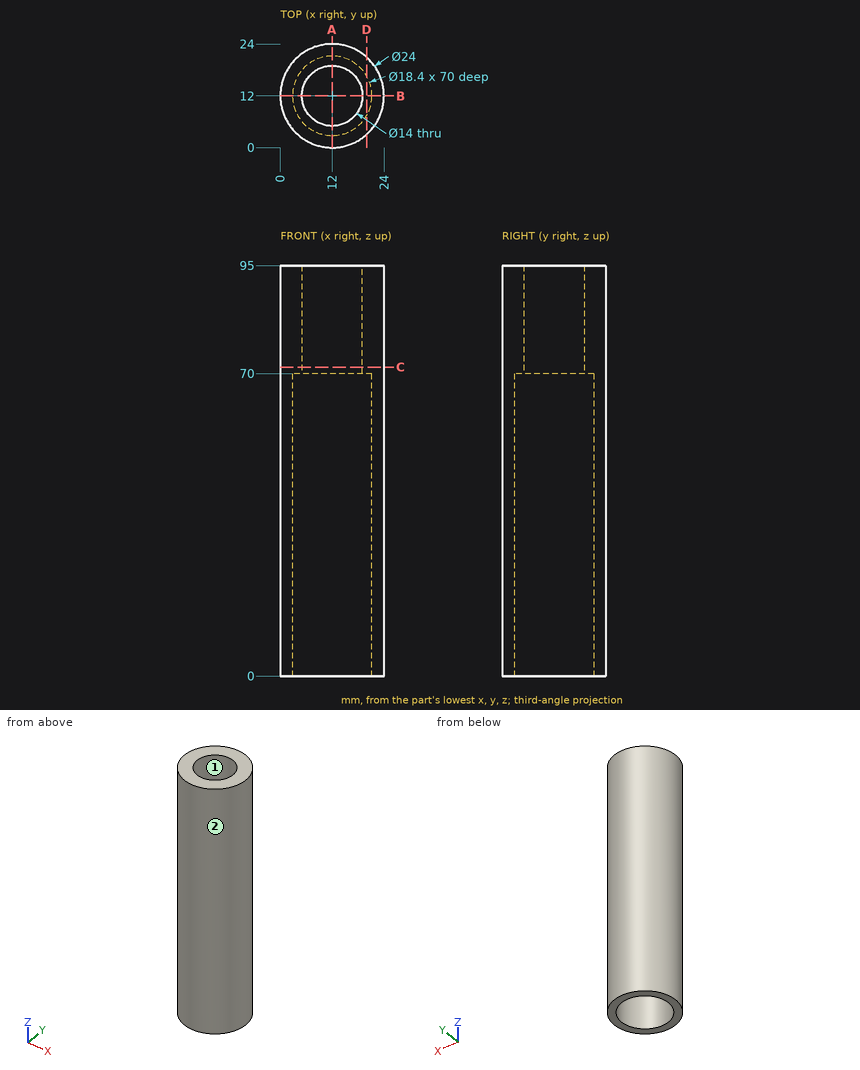
The drawing under review shows one solid part. Ordinate dimensions are in mm from its lowest x, y, z. Give positions to 0.01 mm unless a question says otherwise; leave off trailing zeros. Write each loop counter-clockwise with the first axis right and the second up, starting at its lowest first coordinate (ties: lowest second). Pieces come first, ordered by that corner, then holes. Notation, with made-up numbers: (13.25, 81) -> (48.25, 81) arc R32 ccw to (48.25, 113) -> close; hole circle Ø4 at (9, -10.75). An arc over 180 degrees is marked (long way). Put each result on its own line as item: value.
(1) The part is to be moulded in two halves that separate along Y. For the marked faces 1 and 2, say which applies: pulls with the +Y half, pulls with the -Y half, needs draft (parallel to the pull), parting line crosses it, or undercut.
Results are:
face 1: undercut
face 2: parting line crosses it
(2) We need section A-A, the plane x = 12. Give the boundary of the cut face in (y, z), and give its area (3 significant figures).
Results are:
outline: (0, 0) -> (2.8, 0) -> (2.8, 70) -> (5, 70) -> (5, 95) -> (0, 95) -> close; (19, 70) -> (21.2, 70) -> (21.2, 0) -> (24, 0) -> (24, 95) -> (19, 95) -> close
area: 642 mm²
(3) For pin 1 Ø3 at (x, z) = (10.5, 53.5) entering from -Y; pin 2 Ø1 at (y, z) = (18, 35) entering from -X; pin 3 Ø12.5 at (x, y) = (12, 12) entering from -Z; pin 4 Ø5 at (y, z) = (18.5, 84) entering from -X, all flat-tipped, find the tip position at first contact; note any pin that passes through.
Results are:
pin 1: y = 0
pin 2: x = 1.33
pin 3: through
pin 4: x = 0.69
(4) We need section C-C, the plane z = 71.5. Give the boundary of the cut face in (x, y), and give its area (3 significant figures).
Results are:
outline: circle Ø24 at (12, 12); hole circle Ø14 at (12, 12)
area: 298 mm²
(5) We need section D-D, the plane x = 20. Give the boundary of the cut face in (y, z), and give its area (3 significant figures).
Results are:
outline: (3.06, 0) -> (7.46, 0) -> (7.46, 70) -> (16.54, 70) -> (16.54, 0) -> (20.94, 0) -> (20.94, 95) -> (3.06, 95) -> close
area: 1,060 mm²
(6) To check wall thickness, follow probe 1 along Y at (x, z) = (12, 25.5); probe 2 along Y at (x, z) = (12, 85.5); probe 3 along X at (y, z) = (12.5, 71). State the ranges of each line that lie inside material, in increasing order. Write a range as from..to.
Results are:
probe 1: 0..2.8, 21.2..24
probe 2: 0..5, 19..24
probe 3: 0.01..5.02, 18.98..23.99
